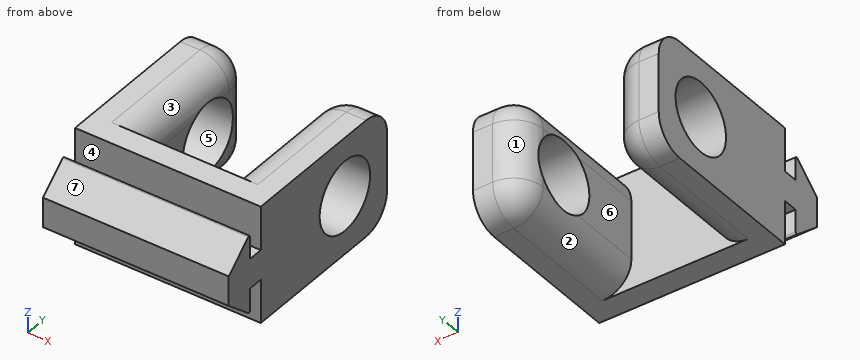
from build123d import *

# Parameters (mm, degrees)
SKETCH10_W              = 2.54
SKETCH10_H              = 5.08
SKETCH10_W_2            = 5.08
SKETCH10_H_2            = 2.54
BOSS_EXTRUDE3_DEPTH     = 31.75
SKETCH11_W              = 20
SKETCH11_H              = 4
BOSS_EXTRUDE4_DEPTH     = 31.75
CUT_EXTRUDE1_DEPTH      = 39.055781427
SKETCH13_W              = 8.375
SKETCH13_H              = 26
BOSS_EXTRUDE5_DEPTH     = 20
CUT_EXTRUDE2_DEPTH      = 50.695881369
CUT_EXTRUDE2_DEPTH_BACK = 50.695881369
SKETCH16_R              = 6
FILLET1_R               = 5


with BuildPart() as part:
    # Sketch10 → Boss-Extrude3 (new body)
    with BuildSketch(Plane(origin=(0, 0, 0), x_dir=(0, 0, -1), z_dir=(1, 0, 0))):
        with Locations((-11.43, 0)):
            Rectangle(SKETCH10_W, SKETCH10_H)
        with BuildLine():
            Line((-5.08, 2.54), (-9.740509205, 6.542688341))
            ThreePointArc((-9.740509205, 6.542688341), (-10.012022021, 6.580814495), (-10.16, 6.35))
            Line((-10.16, 6.35), (-10.16, -6.35))
            ThreePointArc((-10.16, -6.35), (-10.012022021, -6.580814495), (-9.740509205, -6.542688341))
            Line((-9.740509205, -6.542688341), (-5.08, -2.54))
            Line((-5.08, -2.54), (-5.08, 2.54))
        make_face()
        with BuildLine():
            Line((6.35, 10.16), (-6.35, 10.16))
            ThreePointArc((-6.35, 10.16), (-6.580814495, 10.012022021), (-6.542688341, 9.740509205))
            Line((-6.542688341, 9.740509205), (-2.54, 5.08))
            Line((-2.54, 5.08), (2.54, 5.08))
            Line((2.54, 5.08), (6.542688341, 9.740509205))
            ThreePointArc((6.542688341, 9.740509205), (6.580814495, 10.012022021), (6.35, 10.16))
        make_face()
        with Locations((0, 11.43)):
            Rectangle(SKETCH10_W_2, SKETCH10_H_2)
        with BuildLine():
            ThreePointArc((6.542688341, -9.740509205), (6.580814495, -10.012022021), (6.35, -10.16))
            Line((6.35, -10.16), (-6.35, -10.16))
            ThreePointArc((-6.35, -10.16), (-6.580814495, -10.012022021), (-6.542688341, -9.740509205))
            Line((-6.542688341, -9.740509205), (-2.54, -5.08))
            Line((-2.54, -5.08), (2.54, -5.08))
            Line((2.54, -5.08), (6.542688341, -9.740509205))
        make_face()
        with Locations((0, -11.43)):
            Rectangle(SKETCH10_W_2, SKETCH10_H_2)
        with BuildLine():
            Line((5.08, 2.54), (5.08, -2.54))
            Line((5.08, -2.54), (9.740509205, -6.542688341))
            ThreePointArc((9.740509205, -6.542688341), (10.012022021, -6.580814495), (10.16, -6.35))
            Line((10.16, -6.35), (10.16, -2.54))
            Line((10.16, -2.54), (10.16, 2.54))
            Line((10.16, 2.54), (10.16, 6.35))
            ThreePointArc((10.16, 6.35), (10.012022021, 6.580814495), (9.740509205, 6.542688341))
            Line((9.740509205, 6.542688341), (5.08, 2.54))
        make_face()
        with Locations((11.43, 0)):
            Rectangle(SKETCH10_W, SKETCH10_H)
    extrude(amount=-BOSS_EXTRUDE3_DEPTH)

    # Sketch11 → Boss-Extrude4 (add)
    with BuildSketch(Plane(origin=(0, 0, 0), x_dir=(0, 0, -1), z_dir=(1, 0, 0))):
        with Locations((0, 14.7)):
            Rectangle(SKETCH11_W, SKETCH11_H)
    extrude(amount=-BOSS_EXTRUDE4_DEPTH)

    # Sketch12 → Cut-Extrude1 (cut, through all)
    with BuildSketch(Plane.ZY.offset(31.75)):
        Polygon((0, 0), (-15.483602638, 16.020997712), (-15.483602638, -14.964233499), (16.01610749, -14.964233499), (16.01610749, 15.47887645), align=None)
    extrude(amount=-CUT_EXTRUDE1_DEPTH, mode=Mode.SUBTRACT)

    # Sketch13 → Boss-Extrude5 (add, through all)
    with BuildSketch(Plane(origin=(0, 0, -10), x_dir=(-1, 0, 0), z_dir=(0, 0, -1))):
        with Locations((4.1875, 29.7)):
            Rectangle(SKETCH13_W, SKETCH13_H)
        with Locations((27.5625, 29.7)):
            Rectangle(SKETCH13_W, SKETCH13_H)
    extrude(amount=-BOSS_EXTRUDE5_DEPTH)

    # Sketch16 → Cut-Extrude2 (cut, two sides: drawn at the far end of the back side and taken through both)
    with BuildSketch(Plane(origin=(-23.375, 0, 0), x_dir=(0, 0, -1), z_dir=(1, 0, 0)).offset(-CUT_EXTRUDE2_DEPTH_BACK)):
        with Locations(Location((0, 32.7, 0), (0, 0, 90))):
            Circle(SKETCH16_R)
    extrude(amount=CUT_EXTRUDE2_DEPTH + CUT_EXTRUDE2_DEPTH_BACK, mode=Mode.SUBTRACT)

    # Fillet1
    # the kernel refuses this fillet: 5 mm, written as the material it takes off along each edge
    with BuildSketch(Plane(origin=(-3.375, 37.7, 5), x_dir=(0, 1, 0), z_dir=(-1, 0, 0))) as fillet1_piece_1_section:
        Polygon((0, 0), (FILLET1_R * 1.02, 0), (FILLET1_R * 1.02, -FILLET1_R * 1.02), (0, -FILLET1_R * 1.02), align=None)
    fillet1_piece_1 = extrude(amount=FILLET1_R * 1.02, mode=Mode.PRIVATE)
    fillet1_piece_1 = fillet1_piece_1 - Plane(origin=(-3.375, 37.7, 5), x_dir=(0, -0.7071067811865475, -0.7071067811865475), z_dir=(-1, 0, 0)) * Sphere(FILLET1_R, mode=Mode.PRIVATE)
    add(fillet1_piece_1, mode=Mode.SUBTRACT)
    with BuildSketch(Plane(origin=(-3.375, 37.7, -5), x_dir=(0, 0, -1), z_dir=(-1, 0, 0))) as fillet1_piece_2_section:
        Polygon((0, 0), (FILLET1_R * 1.02, 0), (FILLET1_R * 1.02, -FILLET1_R * 1.02), (0, -FILLET1_R * 1.02), align=None)
    fillet1_piece_2 = extrude(amount=FILLET1_R * 1.02, mode=Mode.PRIVATE)
    fillet1_piece_2 = fillet1_piece_2 - Plane(origin=(-3.375, 37.7, -5), x_dir=(0, -0.7071067811865475, 0.7071067811865475), z_dir=(-1, 0, 0)) * Sphere(FILLET1_R, mode=Mode.PRIVATE)
    add(fillet1_piece_2, mode=Mode.SUBTRACT)
    with BuildSketch(Plane(origin=(-28.375, 37.7, 5), x_dir=(1, 0, 0), z_dir=(0, 1, 0))) as fillet1_piece_3_section:
        Polygon((0, 0), (FILLET1_R * 1.02, 0), (FILLET1_R * 1.02, -FILLET1_R * 1.02), (0, -FILLET1_R * 1.02), align=None)
    fillet1_piece_3 = extrude(amount=FILLET1_R * 1.02, mode=Mode.PRIVATE)
    fillet1_piece_3 = fillet1_piece_3 - Plane(origin=(-28.375, 37.7, 5), x_dir=(-0.7071067811865475, 0, -0.7071067811865475), z_dir=(0, 1, 0)) * Sphere(FILLET1_R, mode=Mode.PRIVATE)
    add(fillet1_piece_3, mode=Mode.SUBTRACT)
    with BuildSketch(Plane(origin=(-28.375, 37.7, -5), x_dir=(1, 0, 0), z_dir=(0, 1, 0))) as fillet1_piece_4_section:
        Polygon((0, 0), (FILLET1_R * 1.02, 0), (FILLET1_R * 1.02, FILLET1_R * 1.02), (0, FILLET1_R * 1.02), align=None)
    fillet1_piece_4 = extrude(amount=FILLET1_R * 1.02, mode=Mode.PRIVATE)
    fillet1_piece_4 = fillet1_piece_4 - Plane(origin=(-28.375, 37.7, -5), x_dir=(-0.7071067811865475, 0, 0.7071067811865475), z_dir=(0, 1, 0)) * Sphere(FILLET1_R, mode=Mode.PRIVATE)
    add(fillet1_piece_4, mode=Mode.SUBTRACT)
    with BuildSketch(Plane(origin=(12.5, 42.7, 10), x_dir=(0, 0, -1), z_dir=(-1, 0, 0)), Plane(origin=(12.5, 42.7, -10), x_dir=(0, -1, 0), z_dir=(-1, 0, 0)), Plane(origin=(-28.375, 42.7, -10), x_dir=(0, -1, 0), z_dir=(-1, 0, 0))) as fillet1_piece_5:
        with BuildLine():
            CenterArc((FILLET1_R, FILLET1_R), FILLET1_R, 180, 90)
            Line((0, FILLET1_R), (0, 0))
            Line((0, 0), (FILLET1_R, 0))
        make_face()
    extrude(amount=15.875, mode=Mode.SUBTRACT)
    with BuildSketch(Plane(origin=(-8.375, 37.7, 10), x_dir=(1, 0, 0), z_dir=(0, -1, 0)), Plane(origin=(-23.375, 16.7, 10), x_dir=(-1, 0, 0), z_dir=(0, 1, 0))) as fillet1_piece_6:
        with BuildLine():
            CenterArc((FILLET1_R, -FILLET1_R), FILLET1_R, 90, 90)
            Line((0, -FILLET1_R), (0, 0))
            Line((0, 0), (FILLET1_R, 0))
        make_face()
    extrude(amount=21, mode=Mode.SUBTRACT)
    with BuildSketch(Plane(origin=(-8.375, 42.7, -5), x_dir=(1, 0, 0), z_dir=(0, 0, 1))) as fillet1_piece_7:
        with BuildLine():
            CenterArc((FILLET1_R, -FILLET1_R), FILLET1_R, 90, 90)
            Line((0, -FILLET1_R), (0, 0))
            Line((0, 0), (FILLET1_R, 0))
        make_face()
    extrude(amount=10, mode=Mode.SUBTRACT)
    with BuildSketch(Plane(origin=(-8.375, 37.7, -10), x_dir=(1, 0, 0), z_dir=(0, -1, 0)), Plane(origin=(-23.375, 16.7, -10), x_dir=(-1, 0, 0), z_dir=(0, 1, 0))) as fillet1_piece_8:
        with BuildLine():
            CenterArc((FILLET1_R, FILLET1_R), FILLET1_R, 180, 90)
            Line((0, FILLET1_R), (0, 0))
            Line((0, 0), (FILLET1_R, 0))
        make_face()
    extrude(amount=21, mode=Mode.SUBTRACT)
    with BuildSketch(Plane(origin=(-28.375, 42.7, 10), x_dir=(0, -1, 0), z_dir=(-1, 0, 0))) as fillet1_piece_9:
        with BuildLine():
            CenterArc((FILLET1_R, -FILLET1_R), FILLET1_R, 90, 90)
            Line((0, -FILLET1_R), (0, 0))
            Line((0, 0), (FILLET1_R, 0))
        make_face()
    extrude(amount=15.875, mode=Mode.SUBTRACT)
    with BuildSketch(Plane(origin=(-23.375, 42.7, -5), x_dir=(-1, 0, 0), z_dir=(0, 0, 1))) as fillet1_piece_10:
        with BuildLine():
            CenterArc((FILLET1_R, FILLET1_R), FILLET1_R, 180, 90)
            Line((0, FILLET1_R), (0, 0))
            Line((0, 0), (FILLET1_R, 0))
        make_face()
    extrude(amount=10, mode=Mode.SUBTRACT)


solid = part.part
Geometry: final body of the model. Coordinates: model frame, mm. Face numbers are marked on the shaded views. A direction names the side the tool comes from. Round coordinates to 2 decimals unless told otherwise and drop trailing zeros. Order: outer loops, then holes, each group sorted by start corner. A loop starts at its lowest first (then second) coordinate and runs counter-clockwise, first axis right, second up. Notation, with made-up numbers: (47.5, 26.25) -> (59.5, 26.25) arc R9 ccw to (59.5, 38.25) -> close; hole circle Ø6 at (35, 73.5). An arc over 180 degrees is marked (long way). Put each result on its own line as item: value. Start each with the question number.
Q1. Pull-direction query (Y, two-part tool) for the marked faces 4, 5, 6 and 7; classes: +Y half, -Y half, draft (parallel to the pull), parting line (faces both ways), or undercut.
Q2. Section C-C on x = -17. Return the cut outline in (y, z), and give its area (3 significant figures).
Q3. Section A-A on z = -0.5. Return the cut outline in (x, y) (3 decimals), and give its area (3 significant figures).
Q4. Section B-B on y = 32.7. Return the cut outline in (x, z) (3 decimals), and give its area (3 significant figures).
Q5. Reachability of the marked faces 1, 2 and 3 from +Z, -Z, +X, -X, +Y, -Y: full face, straight path, thin tool, end or side. Return the list, or none.
Q6. Line query: probe 1 along Y at (x, z) = (-29, 0); probe 2 along X at (y, z) = (29, 5) (3 decimals); probe 3 along Y at (x, z) = (-2.5, -3.75). Output: solid intervals per line, ascending.
Q7. First-contact query: pin 1 (3.5 mm diameter, centred on x = -9, z = -5, fed in from -Y); pin 2 (2 mm diameter, centred on x = -9, z = -7.5, fed in from -Y); pin 3 (8 mm diameter, centred on x = -24, z = 1.5, fed in from +Y); pin 4 (9.5 mm diameter, centred on y = 32.7, z = 0, fed in from -X). Flat tips, straight axial feed; report the tip coordinate or a pass-through.
Ans:
1. face 4: undercut
1. face 5: undercut
1. face 6: draft
1. face 7: -Y half
2. outline: (5.08, -2.54) -> (9.74, -6.54) arc R0.25 ccw to (10.16, -6.35) -> (10.16, -2.54) -> (12.7, -2.54) -> (12.7, -10) -> (16.7, -10) -> (16.7, 10) -> (12.7, 10) -> (12.7, 2.54) -> (10.16, 2.54) -> (10.16, 6.35) arc R0.25 ccw to (9.74, 6.54) -> (5.08, 2.54) -> close
2. area: 141 mm2
3. outline: (-31.75, 5.08) -> (0, 5.08) -> (0, 26.721) -> (-8.375, 26.721) -> (-8.375, 16.7) -> (-23.375, 16.7) -> (-23.375, 26.721) -> (-31.75, 26.721) -> close; (-31.75, 38.679) -> (-23.472, 38.679) arc R5 ccw to (-28.375, 42.7) -> (-31.75, 42.7) -> close; (-8.278, 38.679) -> (0, 38.679) -> (0, 42.7) -> (-3.375, 42.7) arc R5 ccw to start
3. area: 593 mm2
4. outline: (-31.75, -10) -> (-28.375, -10) arc R5 ccw to (-23.476, -6) -> (-31.75, -6) -> close; (-31.75, 6) -> (-23.476, 6) arc R5 ccw to (-28.375, 10) -> (-31.75, 10) -> close; (-8.274, -6) arc R5 ccw to (-3.375, -10) -> (0, -10) -> (0, -6) -> close; (-8.274, 6) -> (0, 6) -> (0, 10) -> (-3.375, 10) arc R5 ccw to start
4. area: 113 mm2
5. face 1: +Z, -Z, +Y
5. face 2: -Z, +Y
5. face 3: +Z, +Y
6. probe 1: y = 5.08 to 26.7, 38.7 to 42.7
6. probe 2: x = -31.75 to -23.375, -8.375 to 0
6. probe 3: y = 6.49 to 10.16, 12.7 to 28.02, 37.38 to 42.7
7. pin 1: stops at y = 5.91
7. pin 2: stops at y = 9.69
7. pin 3: stops at y = 42.69
7. pin 4: passes through
